Input: part model. Units: mm. Frame: model coordinates. A direction names the side the tool comes from. Coordinates: 2 decimals unless noted, no trailing zeros. Loops run counter-clockwise (first coordinate to the right, second up) from the corner with the lowest first, then second, coordinate; pieces in that order, holes last. Notation, with made-up numbers: (7, -5.5) - (60, -5.5) arc R18 ccw to (60, 25.5) - close; hole circle Ø6 at (64, -22.5). An arc over 180 degrees is marked (long way). Use one line per item in the form item = value.
from build123d import *

# Parameters (mm, degrees)
ESQUISSE2_R        = 9.25
ESQUISSE2_R_2      = 7.25
BOSS_EXTRU_1_DEPTH = 45
ESQUISSE5_R        = 1.5


with BuildPart() as part:
    # Esquisse2 → Boss.-Extru.1 (new, symmetric)
    with BuildSketch(Plane.XY):
        with Locations(Location((0, 0, 0), (0, 0, 180))):
            Circle(ESQUISSE2_R)
        with Locations(Location((0, 0, 0), (0, 0, 180))):
            Circle(ESQUISSE2_R_2, mode=Mode.SUBTRACT)
    extrude(amount=BOSS_EXTRU_1_DEPTH, both=True)

    # Esquisse3 → Révolution1 (revolve)
    with BuildSketch(Plane(origin=(0, 0, 0), x_dir=(1, 0, 0), z_dir=(0, 1, 0))):
        with BuildLine():
            Line((-5.25, 49), (0, 49))
            Line((0, 49), (0, 45))
            Line((0, 45), (-9.25, 45))
            ThreePointArc((-9.25, 45), (-8.078427125, 47.828427125), (-5.25, 49))
        make_face()
    revolve(axis=Axis((0, 0, -49), (0, 0, 1)))

    # Balayage3: sweep along a path in Esquisse6
    with BuildLine(Plane(origin=(0, 0, 0), x_dir=(1, 0, 0), z_dir=(0, 1, 0))) as balayage3_path:
        Line((-4.25, 45), (-4.25, 59.75))
        ThreePointArc((-4.25, 59.75), (0, 64), (4.25, 59.75))
    # Esquisse5 → Balayage3 (sweep)
    with BuildSketch(Plane(origin=(0, 0, 0), x_dir=(0, 0, -1), z_dir=(1, 0, 0))):
        with Locations((65.5, 0)):
            Circle(ESQUISSE5_R)
    sweep(path=balayage3_path.line)


solid = part.part
Q1. Cut plane A-A, the plane x = 0. Return loops of the section in (y, z).
Check values:
outline = (-9.25, -45) arc R4 ccw to (-5.25, -49) - (5.25, -49) arc R4 ccw to (9.25, -45) - (9.25, 45) - (7.25, 45) - (7.25, -45) - (-7.25, -45) - (-7.25, 45) - (-9.25, 45) - close; circle Ø3 at (0, -65.5)
Q2. Pull-direction query (Z, two-part tool) for faces 1 (the flat face through (0, 0, -49)), 2 (the flat face through (0, 0, -45)), 3 (the cylindrical face through (-4.268, 8.206, 0.63)); classes: pulls with the +Z half, pulls with the -Z half, needs draft (parallel to the pull), parting line crosses it, or undercut.
Check values:
face_1 = undercut
face_2 = pulls with the +Z half
face_3 = needs draft
Q3. Ray query, line 1 along Y through (x, z) = (0, 6.5); line 2 along Y through (x, z) = (-5, 24); line 3 along Z through (x, y) = (3, -3.5). Return the intervals inside material, ascending. Write a range as [from, to].
Check values:
line_1 = [-9.25, -7.25], [7.25, 9.25]
line_2 = [-7.78, -5.25], [5.25, 7.78]
line_3 = [-49, -45]
Q4. Cut plane D-D, the plane z = -58.5. Return loops of the section in (x, y).
Check values:
outline = circle Ø3 at (-5.75, 0)
Q5. Cut plane C-C, the plane z = 0. Return loops of the section in (x, y).
Check values:
outline = circle Ø18.5 at (0, 0); hole circle Ø14.5 at (0, 0)
Q6. Set-up query: faces 4 (the cylindrical face through (-4.56, -0.91, -54.19)), 5 (the cylindrical face through (-3.35, 6.43, -0.63)), 6 (the flat face through (6, 0, -59.75)). Return all of +Z, -Z, +X, -X, +Y, -Y with unobstructed straight access to the full face (end or side cutting, diameter ignored); none if empty.
Check values:
face_4 = none
face_5 = +Z
face_6 = +X, +Y, -Y
Q7. Cut plane B-B, the plane y = 0. Return loops of the section in (x, z).
Check values:
outline = (-9.25, -45) arc R4 ccw to (-7.25, -48.46) - (-7.25, -59.75) arc R7.25 ccw to (7.25, -59.75) - (4.25, -59.75) arc R4.25 cw to (-4.25, -59.75) - (-4.25, -49) - (5.25, -49) arc R4 ccw to (9.25, -45) - (9.25, 45) - (7.25, 45) - (7.25, -45) - (-7.25, -45) - (-7.25, 45) - (-9.25, 45) - close
Q8. First-contact query: P1, Ø6, axis at x = 6.5, z = 17, coming from the -Y side; P2, Ø3, axis at x = -1.5, y = -4, coming from the +Z side; P3, Ø5, axis at y = 7, z = -8.5, coming from the +X side. Flat tips, straight axial feed; report the tip coordinate or a pass-through.
Check values:
P1 = -8.56
P2 = -45
P3 = 8.08
